Check sheet for the drawn part. Datum: minimum x, y, z corner. Units: mm. Give positions to 0.01 mm unless a question says otherwise; leave off trailing zeros. Write each loop counter-clockwise with the first axis right and the second up, starting at its lowest first coordinate (ties: lowest second). Pieces come first, ordered by that corner, then holes. Notation, with made-up numbers: (0.25, -2.75) - (9.25, -2.75) arc R25 ccw to (9.25, 24.25) - close; hole circle Ø10 at (-33.75, -13.5). An arc over 180 degrees is marked (long way). Answer as a JSON object with one key per item and string values. Group by question number.
Item 1: Sectioned sample at B-B, the plane z = 160. Record the boundary of the cut face in (x, y).
Item 2: Scan lines: line 1 along X through (y, z) = (8.25, 160); line 2 along Z through (x, y) = (37.5, 2.75); line 3 along X through (y, z) = (9.25, 180.5). Record each from-to range of solid material in increasing order. Write a range as [from, to].
Item 3: Sectioned sample at A-A, the plane x = 37. Record the boundary of the cut face in (y, z), and give its area (3 significant figures).
Item 4: Sectioned sample at C-C, the plane y = 2.5. Record the boundary of the cut face in (x, z), and give its area (3 significant figures).
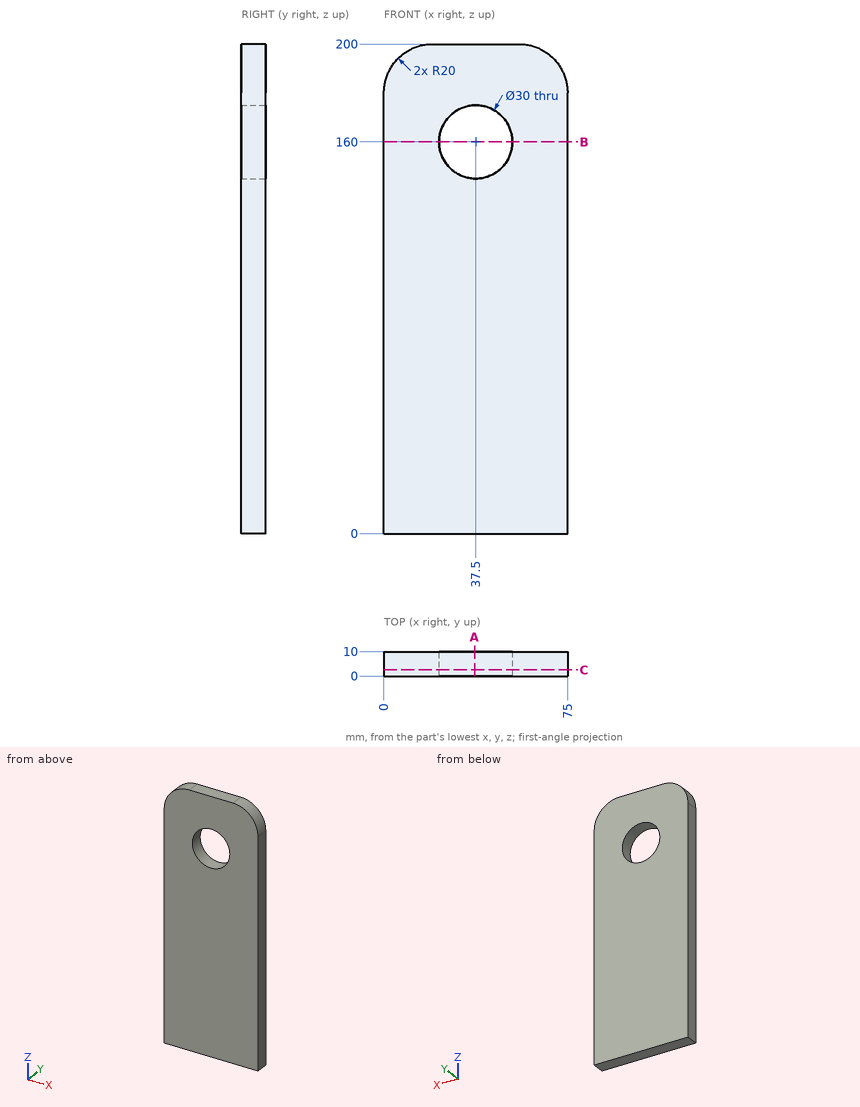
Geometry check:
{
 "1": {"outline": "(0, 0) - (22.5, 0) - (22.5, 10) - (0, 10) - close; (52.5, 0) - (75, 0) - (75, 10) - (52.5, 10) - close"},
 "2": {"line 1": "[0, 22.5], [52.5, 75]", "line 2": "[0, 145], [175, 200]", "line 3": "[0.01, 74.99]"},
 "3": {"outline": "(0, 0) - (10, 0) - (10, 145.01) - (0, 145.01) - close; (0, 174.99) - (10, 174.99) - (10, 200) - (0, 200) - close", "area": "1,700 mm^2"},
 "4": {"outline": "(0, 0) - (75, 0) - (75, 180) arc R20 ccw to (55, 200) - (20, 200) arc R20 ccw to (0, 180) - close; hole circle Ø30 at (37.5, 160)", "area": "14,100 mm^2"}
}
